Autodesk Inventor part; units mm, degrees
ref_plane "YZ Plane" through (0, 0, 0) normal (1, 0, 0) x (0, 1, 0)
ref_plane "XZ Plane" through (0, 0, 0) normal (0, 1, 0) x (-1, 0, 0)
ref_plane "XY Plane" through (0, 0, 0) normal (0, 0, 1) x (1, 0, 0)
sketch "草图1" plane through (0, 0, 0) normal (0, 0, 1) x (1, 0, 0)
  circle A0 centre (0, 0) radius 10
  dimension "d0" = 20
extrude "拉伸1" add sketch "草图1" along normal blind 2
sketch "草图2" plane through (0, 0, 2) normal (0, 0, 1) x (1, 0, 0)
  line L0 (4.3301, -7.5) -> (-4.3301, -7.5)
  line L1 (-4.3301, -7.5) -> (-8.6603, 0)
  line L2 (-8.6603, 0) -> (-4.3301, 7.5)
  line L3 (-4.3301, 7.5) -> (4.3301, 7.5)
  line L4 (4.3301, 7.5) -> (8.6603, 0)
  line L5 (8.6603, 0) -> (4.3301, -7.5)
  line L6 (0, 0) -> (0, 2.6407)
  point P0 (0, 7.5)
  dimension "d3" = 2.6407
  dimension "d4" = 15
extrude "拉伸2" add sketch "草图2" along normal blind 8
fillet "圆角1" radius 0.5 13 edges at (-10, 0, 2) (0, 7.5, 10) (4.3301, 7.5, 6) (-4.3301, 7.5, 6) (-6.4952, 3.75, 10) (6.4952, 3.75, 10) (-6.4952, -3.75, 10) (0, -7.5, 10) (6.4952, -3.75, 10) (8.6603, 0, 6) (4.3301, -7.5, 6) (-4.3301, -7.5, 6) (-8.6603, 0, 6)
sketch "草图3" plane through (0, 0, 0) normal (0, 0, -1) x (-1, 0, 0)
  circle A0 centre (0, 0) radius 5
  dimension "d8" = 10
extrude "拉伸3" cut sketch "草图3" against normal through all
thread "螺纹1"
properties part number "托带轮固定螺丝"
The listing builds one solid part. Answer for the finished solid, in the listing's coordinates (mm). A direction names the side the tool comes from. Give positions to 0.01 mm unless a question says otherwise; leave off trailing zeros. Order: outer loops, then holes, each group sorted by start corner. A loop starts at its lowest first (then second) coordinate and runs counter-clockwise, first axis right, second up. Notation, with made-up numbers: (-15.75, -10) - (31.25, -10) arc R22 ccw to (31.25, 28) - close; hole circle Ø3 at (60, -11.75). An arc over 180 degrees is marked (long way). One line per item, written item: value. Start each with the question number.
1) A cutting plane is placed at A-A on x = 0. Give the vertices of the cut face in (y, z).
2) A tool of negligible diameter and unlimited length cuts with its end or side. For faces 1 (the face through (-6.523, 3.701, 5.698)), 2 (the face through (6.467, 3.799, 5.698)), 3 (the face through (0, -7.5, 6)), 4 (the face through (6.523, -3.701, 5.698)), 5 (the face through (0, -8, 2)), from which of +Z, -Z, +X, -X, +Y, -Y can it reach the whole face along a straight path? Write none if from no direction.
3) A cutting plane is placed at C-C on z = 9.75. Give the vertices of the cut face in (x, y).
4) Given pin 1 Ø5 at (x, z) = (6, 8) entering from -Y; pin 2 Ø4 at (x, z) = (1, 6.5) entering from +Y; pin 3 Ø1.5 at (y, z) = (8, 6) entering from +X, each flat-ended and moving along its own axis, determine where each tip first touches the part or whether it passes through.
5) A cutting plane is placed at B-B on z = 5. Give the vertices of the cut face in (x, y).
6) Find the intervals of material crossed by L1, parallel to Y at x = 0, z = 2.5; L2, parallel to X at y = -0.25, z = 3; L3, parallel to Z at x = 4.75, y = -7.75, in increasing order.
7) The mould has two halves that part along X. Classify faces 6 (the face through (-6.467, -3.799, 5.698)), 7 (the face through (6.34, -3.73, 9.85)), 8 (the face through (1.08, -4.88, 4.93)), 9 (the face through (0, 7.5, 6)): released by +X, released by -X, zero draft, split by the parting line, or undercut.
Answer sheet:
1. outline: (-10, 0) - (-5, 0) - (-5, 10) - (-7, 10) arc R0.5 ccw to (-7.5, 9.5) - (-7.5, 2) - (-9.5, 2) arc R0.5 ccw to (-10, 1.5) - close; (5, 0) - (10, 0) - (10, 1.5) arc R0.5 ccw to (9.5, 2) - (7.5, 2) - (7.5, 9.5) arc R0.5 ccw to (7, 10) - (5, 10) - close
2. face 1: +Z, -X, +Y
2. face 2: +Z, +X, +Y
2. face 3: +Z, +X, -X, -Y
2. face 4: +Z, +X, -Y
2. face 5: +Z
3. outline: (-8.46, -0.22) - (-4.42, -7.22) arc R0.43 ccw to (-4.04, -7.43) - (4.04, -7.43) arc R0.43 ccw to (4.42, -7.22) - (8.46, -0.22) arc R0.43 ccw to (8.46, 0.22) - (4.42, 7.22) arc R0.43 ccw to (4.04, 7.43) - (-4.04, 7.43) arc R0.43 ccw to (-4.42, 7.22) - (-8.46, 0.22) arc R0.43 ccw to start; hole circle Ø10 at (0, 0)
4. pin 1: stops at y = -7.5
4. pin 2: stops at y = 7.5
4. pin 3: stops at x = 4.47
5. outline: (-8.52, -0.25) - (-4.47, -7.25) arc R0.5 ccw to (-4.04, -7.5) - (4.04, -7.5) arc R0.5 ccw to (4.47, -7.25) - (8.52, -0.25) arc R0.5 ccw to (8.52, 0.25) - (4.47, 7.25) arc R0.5 ccw to (4.04, 7.5) - (-4.04, 7.5) arc R0.5 ccw to (-4.47, 7.25) - (-8.52, 0.25) arc R0.5 ccw to start; hole circle Ø10 at (0, 0)
6. L1: y = -7.5 to -5, 5 to 7.5
6. L2: x = -8.52 to -4.99, 4.99 to 8.52
6. L3: z = 0 to 2
7. face 6: released by -X
7. face 7: released by +X
7. face 8: undercut
7. face 9: zero draft
